The listing builds one solid part. Answer for the finished solid, in the listing's coordinates (mm). A direction names the side the tool comes from. Give positions to 0.01 mm unless a question says otherwise; leave off trailing zeros. Write each loop counter-clockwise with the first axis right and the second up, starting at its lowest first coordinate (ties: lowest second). Pieces come first, ordered by that corner, then holes. Notation, with made-up numbers: (-22, -31.75) - (23, -31.75) arc R8 cw to (23, -25.75) - close; hole circle Ø4 at (-1, 36). An arc over 180 degrees is marked (long way). Use a Markdown table: item, result. Add a question column.
from build123d import *

# Parameters (mm, degrees)
F0_W     = 47.95
F0_H     = 15.88
F0_R     = 2.46
F1_DEPTH = 3.12
F3_R     = 2.465
F4_DEPTH = 2.28
F5_W     = 44.987634
F5_H     = 13.142811
F6_DEPTH = 1.91
F7_R     = 3.285
F8_DEPTH = 1.93


with BuildPart() as f1:
    # F0 (on Front) → F1 (new body)
    with BuildSketch(Plane.XZ):
        with Locations((-62.765208, 37.205729)):
            Rectangle(F0_W, F0_H)
        with Locations((-83.495483, 34.202196)):
            Circle(F0_R, mode=Mode.SUBTRACT)
        with Locations((-76.453662, 34.202196)):
            Circle(F0_R, mode=Mode.SUBTRACT)
        with Locations((-69.286012, 34.202196)):
            Circle(F0_R, mode=Mode.SUBTRACT)
        with Locations((-83.495483, 41.639235)):
            Circle(F0_R, mode=Mode.SUBTRACT)
        with Locations((-76.453662, 41.639235)):
            Circle(F0_R, mode=Mode.SUBTRACT)
        with Locations((-69.286012, 41.639235)):
            Circle(F0_R, mode=Mode.SUBTRACT)
        with Locations((-61.757147, 34.202196)):
            Circle(F0_R, mode=Mode.SUBTRACT)
        with Locations((-53.794272, 34.202196)):
            Circle(F0_R, mode=Mode.SUBTRACT)
        with Locations((-44.286012, 34.202196)):
            Circle(F0_R, mode=Mode.SUBTRACT)
        with Locations((-62.190687, 41.639235)):
            Circle(F0_R, mode=Mode.SUBTRACT)
        with Locations((-53.676993, 41.639235)):
            Circle(F0_R, mode=Mode.SUBTRACT)
        with Locations((-44.286012, 41.639235)):
            Circle(F0_R, mode=Mode.SUBTRACT)
        with Locations((-83.495483, 41.639235)):
            Circle(F0_R)
        with Locations((-83.495483, 34.202196)):
            Circle(F0_R)
        with Locations((-76.453662, 34.202196)):
            Circle(F0_R)
        with Locations((-76.453662, 41.639235)):
            Circle(F0_R)
        with Locations((-69.286012, 34.202196)):
            Circle(F0_R)
        with Locations((-69.286012, 41.639235)):
            Circle(F0_R)
        with Locations((-61.757147, 34.202196)):
            Circle(F0_R)
        with Locations((-62.190687, 41.639235)):
            Circle(F0_R)
        with Locations((-53.794272, 34.202196)):
            Circle(F0_R)
        with Locations((-53.676993, 41.639235)):
            Circle(F0_R)
        with Locations((-44.286012, 34.202196)):
            Circle(F0_R)
        with Locations((-44.286012, 41.639235)):
            Circle(F0_R)
    extrude(amount=F1_DEPTH)

    # F3 (on face) → F4 (join)
    with BuildSketch(Plane.XZ.offset(3.12)):
        with BuildLine():
            ThreePointArc((-85.161299, 39.95467), (-82.693921, 37.494436), (-80.231304, 39.959435))
            ThreePointArc((-80.231304, 39.959435), (-82.698686, 42.424434), (-85.161299, 39.95467))
        make_face()
        with Locations((-82.696304, 33.589986)):
            Circle(F3_R)
        with Locations((-76.319206, 39.959435)):
            Circle(F3_R)
        with Locations((-76.319206, 33.553134)):
            Circle(F3_R)
        with Locations((-69.843043, 39.959435)):
            Circle(F3_R)
        with Locations((-63.444085, 39.959435)):
            Circle(F3_R)
        with Locations((-55.449564, 39.959435)):
            Circle(F3_R)
        with Locations((-70.081018, 33.553134)):
            Circle(F3_R)
        with Locations((-63.444085, 33.553134)):
            Circle(F3_R)
        with Locations((-55.449564, 33.553134)):
            Circle(F3_R)
        with Locations((-47.453236, 33.553134)):
            Circle(F3_R)
        with Locations((-47.453236, 39.959435)):
            Circle(F3_R)
    extrude(amount=F4_DEPTH)

    # F5 (on face) → F6 (cut)
    with BuildSketch(Plane(origin=(0, 0, 0), x_dir=(-1, 0, 0), z_dir=(0, 1, 0))):
        with Locations((62.636159, 37.369034)):
            Rectangle(F5_W, F5_H)
    extrude(amount=-F6_DEPTH, mode=Mode.SUBTRACT)

    # F7 (on face) → F8 (join)
    with BuildSketch(Plane(origin=(0, -1.91, 0), x_dir=(-1, 0, 0), z_dir=(0, 1, 0))):
        with Locations((46.452342, 37.369034)):
            Circle(F7_R)
        with Locations((53.832342, 37.369034)):
            Circle(F7_R)
        with Locations((61.212342, 37.369034)):
            Circle(F7_R)
        with Locations((68.592342, 37.369034)):
            Circle(F7_R)
        with Locations((75.972342, 37.369034)):
            Circle(F7_R)
    extrude(amount=F8_DEPTH)


solid = f1.part
1. The part is cut by section C-C (x = -77). Give the vertices of the cut face in (y, z).
2. Consider L1, parallel to X at y = -3.8, z = 33.5; L2, parallel to X at y = -3.25, z = 32; L3, parallel to X at y = -0.25, z = 31.5. Determine where each line is inside the solid, lowest interval first. Write a range as [from, to].
3. The part is cut by section B-B (y = -4.3). Count the separate pieces of the cut face and the enclosed holes in it, and give its area (3 significant figures).
4. For a pull along Z with two mould halves and no side action, classify faces 1 (the flat face through (-47, -5.4, 40)), 2 (the flat face through (-63, -2, 45.146)), 3 (the cylindrical face through (-67.804, -4.244, 32.609)) as released by +Z, released by -Z, zero draft, split by the parting line, or undercut.
5. Given P1, Ø8, axis at x = -60.5, z = 33.5, coming from the -Y side; P2, Ø1, axis at x = -77.5, z = 33, coming from the +Y side, each flat-ended and moving along its own axis, determine where each tip first touches the part or whether it passes through.
6. The part is cut by section A-A (y = -1.5). Give the vertices of the cut face in (x, z) (3 decimals), and give its area (3 significant figures).
7. Which of the six approach directions +Z, -Z, +X, -X, +Y, -Y give full straight-line access (tool end or side, diameter ignored) to faces 4 (the flat face through (-83, -5.4, 34)), 5 (the flat face through (-62, -1.91, 42)), 6 (the cylindrical face through (-68.71, -4.24, 37.77))?
Check values:
| question | item | result |
|---|---|---|
| 1 | outline | (-5.4, 31.18) - (-3.12, 31.18) - (-3.12, 29.27) - (0, 29.27) - (0, 30.8) - (-1.91, 30.8) - (-1.91, 34.25) - (0.02, 34.25) - (0.02, 40.49) - (-1.91, 40.49) - (-1.91, 43.94) - (0, 43.94) - (0, 45.15) - (-3.12, 45.15) - (-3.12, 42.33) - (-5.4, 42.33) - (-5.4, 37.59) - (-3.12, 37.59) - (-3.12, 35.92) - (-5.4, 35.92) - close |
| 2 | L1 | x = [-85.16, -80.23], [-78.78, -73.85], [-72.55, -67.62], [-65.91, -60.98], [-57.91, -52.99], [-49.92, -44.99] |
| 2 | L2 | x = [-84.58, -80.81], [-78.23, -74.41], [-72, -68.17], [-65.36, -61.53], [-57.36, -53.54], [-49.37, -45.54] |
| 2 | L3 | x = [-86.74, -85.13], [-40.14, -38.79] |
| 3 | separate pieces | 12 |
| 3 | enclosed holes | 0 |
| 3 | area | 229 mm2 |
| 4 | face 1 | zero draft |
| 4 | face 2 | released by +Z |
| 4 | face 3 | undercut |
| 5 | P1 | stops at y = -5.4 |
| 5 | P2 | stops at y = -1.91 |
| 6 | outline | (-86.74, 29.266) - (-38.79, 29.266) - (-38.79, 45.146) - (-86.74, 45.146) - close; circle Ø6.57 at (-75.972, 37.369); circle Ø6.57 at (-68.592, 37.369); circle Ø6.57 at (-61.212, 37.369); circle Ø6.57 at (-53.832, 37.369); circle Ø6.57 at (-46.452, 37.369); hole (-85.13, 30.798) - (-40.142, 30.798) - (-40.142, 43.94) - (-85.13, 43.94) - close |
| 6 | area | 340 mm2 |
| 7 | face 4 | +Z, -Z, +X, -X, -Y |
| 7 | face 5 | +Y |
| 7 | face 6 | -Y |
